```python
from build123d import *

# Parameters (mm, degrees)
SKETCH2_W           = 136.932578545
SKETCH2_H           = 134.741657288
CUT_EXTRUDE1_DEPTH  = 41
SKETCH3_W           = 157.433341732
SKETCH3_H           = 136.306601043
CUT_EXTRUDE2_DEPTH  = 41
CUT_EXTRUDE3_DEPTH  = 41
CUT_EXTRUDE4_START  = -3
SKETCH8_R           = 3.5
CUT_EXTRUDE4_DEPTH  = 43
CUT_EXTRUDE5_DEPTH  = 24
CIRPATTERN1_COUNT   = 6
CIRPATTERN2_COUNT   = 3
BOSS_EXTRUDE1_DEPTH = 4
CUT_EXTRUDE6_DEPTH  = 5
SKETCH12_R          = 5
CUT_EXTRUDE7_DEPTH  = 45.0000001


with BuildPart() as part:
    # Sketch1 → Revolve1 (revolve)
    with BuildSketch(Plane.XY):
        with BuildLine():
            Line((0, 0), (0, 60))
            ThreePointArc((0, 60), (-60, 0), (0, -60))
            Line((0, -60), (0, 0))
        make_face()
    revolve(axis=Axis((0, 0, 0), (0, 1, 0)))

    # Sketch2 → Cut-Extrude1 (cut, through all)
    with BuildSketch(Plane(origin=(0, 20, 0), x_dir=(1, 0, 0), z_dir=(0, 1, 0))):
        with Locations((2.269168444, -1.72143813)):
            Rectangle(SKETCH2_W, SKETCH2_H)
    extrude(amount=CUT_EXTRUDE1_DEPTH, mode=Mode.SUBTRACT)

    # Sketch3 → Cut-Extrude2 (cut, through all)
    with BuildSketch(Plane(origin=(0, -20, 0), x_dir=(1, 0, 0), z_dir=(0, 1, 0))):
        with Locations((3.912359387, -2.503910008)):
            Rectangle(SKETCH3_W, SKETCH3_H)
    extrude(amount=-CUT_EXTRUDE2_DEPTH, mode=Mode.SUBTRACT)

    # Sketch7 → Cut-Extrude3 (cut, through all)
    with BuildSketch(Plane(origin=(0, 20, 0), x_dir=(1, 0, 0), z_dir=(0, 1, 0))):
        with BuildLine():
            Line((48.989794856, 16), (63.030663811, 16))
            Line((63.030663811, 16), (63.030663811, -16))
            Line((63.030663811, -16), (48.989794856, -16))
            ThreePointArc((48.989794856, -16), (32.989794856, 0), (48.989794856, 16))
        make_face()
    cut_extrude3 = extrude(amount=-CUT_EXTRUDE3_DEPTH, mode=Mode.SUBTRACT)

    # Sketch8 → Cut-Extrude4 (cut)
    with BuildSketch(Plane.XY.offset(-16).offset(CUT_EXTRUDE4_START)):
        with Locations((48, 0)):
            Circle(SKETCH8_R)
    cut_extrude4 = extrude(amount=CUT_EXTRUDE4_DEPTH, mode=Mode.SUBTRACT)

    # Sketch9 → Cut-Extrude5 (cut)
    with BuildSketch(Plane.XY):
        with BuildLine():
            Line((45.422340515, 2.36762995), (57.946221285, 16.002488752))
            Line((57.946221285, 16.002488752), (63.101540255, 11.267228853))
            Line((63.101540255, 11.267228853), (50.577659485, -2.36762995))
            ThreePointArc((50.577659485, -2.36762995), (45.63237005, -2.577659485), (45.422340515, 2.36762995))
        make_face()
    cut_extrude5 = extrude(amount=CUT_EXTRUDE5_DEPTH, mode=Mode.SUBTRACT)

    # CirPattern1: Cut-Extrude3 ×6 about axis
    cirpattern1_axis = Axis((0, 0, 0), (0, 1, 0))
    for i in range(1, CIRPATTERN1_COUNT):
        add(cut_extrude3.rotate(cirpattern1_axis, i * 360 / CIRPATTERN1_COUNT), mode=Mode.SUBTRACT)

    # CirPattern2: Cut-Extrude4, Cut-Extrude5 ×3 about axis
    cirpattern2_axis = Axis((0, 0, 0), (0, 1, 0))
    for i in range(1, CIRPATTERN2_COUNT):
        add(cut_extrude4.rotate(cirpattern2_axis, i * 360 / CIRPATTERN2_COUNT), mode=Mode.SUBTRACT)
        add(cut_extrude5.rotate(cirpattern2_axis, i * 360 / CIRPATTERN2_COUNT), mode=Mode.SUBTRACT)

    # Sketch10 → Boss-Extrude1 (add)
    with BuildSketch(Plane(origin=(0, 20, 0), x_dir=(1, 0, 0), z_dir=(0, 1, 0))):
        Polygon((27, -15.588457268), (27, 15.588457268), (0, 31.176914536), (-27, 15.588457268), (-27, -15.588457268), (0, -31.176914536), align=None)
    extrude(amount=BOSS_EXTRUDE1_DEPTH)

    # Sketch11 → Cut-Extrude6 (cut)
    with BuildSketch(Plane.XZ.offset(20)):
        Polygon((27, -15.588457268), (27, 15.588457268), (0, 31.176914536), (-27, 15.588457268), (-27, -15.588457268), (0, -31.176914536), align=None)
    extrude(amount=-CUT_EXTRUDE6_DEPTH, mode=Mode.SUBTRACT)

    # Sketch12 → Cut-Extrude7 (cut, through all)
    with BuildSketch(Plane(origin=(0, 24, 0), x_dir=(1, 0, 0), z_dir=(0, 1, 0))):
        Circle(SKETCH12_R)
    extrude(amount=-CUT_EXTRUDE7_DEPTH, mode=Mode.SUBTRACT)


solid = part.part
```
Geometry check sheet. Reference: the model listing, model coordinates, mm. A direction names the side the tool comes from. Round coordinates to 2 decimals unless told otherwise and drop trailing zeros. Order: outer loops, then holes, each group sorted by start corner. A loop starts at its lowest first (then second) coordinate and runs counter-clockwise, first axis right, second up. Notation, with made-up numbers: (64.25, -20.75) -> (110.25, -20.75) arc R19 ccw to (110.25, -7.75) -> close; hole circle Ø4 at (76, 45.25). An arc over 180 degrees is marked (long way). Return JSON: item names as keys, results as strings. Group by question number.
Q1. Material ranges on probe 1 along X at (y, z) = (10, 0); probe 2 along X at (y, z) = (-3, -30); probe 3 along Y at (x, z) = (48, -16.6), recorded low to high. Write a range as from..to.
Q2. Gauge pin test, flat ends, axial feed: pin 1 (1.5 mm diameter, centred on y = -15, z = 6, fed in from -X); pin 2 (12 mm diameter, centred on y = 12, z = 1, fed in from -X); pin 3 (1.5 mm diameter, centred on x = -45, y = -11, fed in from +Z). Record the tip position at first contact, or that the pin passes through.
Q3. Section check A-A, the plane z = 0. Record the boundary of the cut face in (x, y), plus the area to 3 significant figures.
Q4. Section check C-C, the plane z = 44.5. Record the boundary of the cut face in (x, y), plus the area to 3 significant figures.
Q5. Tool access check on faces 4 (the flat face through (50.69, 8.1, 19.74)), 5 (the flat face through (27, -18, 0)), 6 (the cylindrical face through (16.8, 0.3, -28.4)), 7 (the flat face through (-12.05, 14.75, -52.87)), 8 (the flat face through (12.326, 0.28, -53.349)). Record the directions out of +Z, -Z, +X, -X, +Y, -Y that give a thin tool (end or side, any length) a straight path to the whole face; none if there is none.
Q6. Release check for a two-part mould opening along Z. For faces 1 (the flat face through (-40.53, 0.28, -38.2)), 2 (the cylindrical face through (-1.08, 4.77, 4.88)), 3 (the flat face through (-12, 20, -25)) record: released by +Z, released by -Z, zero draft, split by the parting line, or undercut.
Numbers:
{
 "1": {"probe 1": "-32.99..-5, 5..32.99", "probe 2": "-51.87..-34.57, -14.42..14.42, 34.57..51.87", "probe 3": "-20..-3.5, 3.5..20"},
 "2": {"pin 1": "x = -34.48", "pin 2": "x = -34.6", "pin 3": "z = 39.02"},
 "3": {"outline": "(-32.99, -20) -> (-27, -20) -> (-27, -15) -> (-5, -15) -> (-5, 24) -> (-27, 24) -> (-27, 20) -> (-32.99, 20) -> close; (5, -15) -> (27, -15) -> (27, -20) -> (32.99, -20) -> (32.99, 20) -> (27, 20) -> (27, 24) -> (5, 24) -> close", "area": "2,200 mm^2"},
 "4": {"outline": "(-8.63, -20) -> (8.63, -20) -> (8.63, 20) -> (-8.63, 20) -> close", "area": "690 mm^2"},
 "5": {"face 4": "none", "face 5": "-Y", "face 6": "+Y, -Y", "face 7": "-X, +Y, -Y", "face 8": "+X, +Y, -Y"},
 "6": {"face 1": "released by -Z", "face 2": "undercut", "face 3": "zero draft"}
}
